from build123d import *

# Parameters (mm, degrees)
F0_W     = 127.9261372983
F0_H     = 87.7036768943
F1_DEPTH = 45.72
F2_R     = 17.7920916597
F3_DEPTH = 45.72
F4_W     = 127.9261372983
F4_H     = 45.72
F4_R     = 16.3569276355
F5_DEPTH = 130.048
F6_DEPTH = 25.4
F7_DEPTH = 104.394


with BuildPart() as f1:
    # F0 (on Top) → F1 (new body)
    with BuildSketch(Plane.XY):
        with Locations((-2.9164496809, -12.6540614292)):
            Rectangle(F0_W, F0_H)
    extrude(amount=F1_DEPTH)

    # F2 (on face) → F3 (cut)
    with BuildSketch(Plane.XY.offset(45.72)):
        with Locations((-40.4178053141, 0)):
            Circle(F2_R)
    extrude(amount=-F3_DEPTH, mode=Mode.SUBTRACT)

    # F4 (on face) → F5 (join)
    with BuildSketch(Plane(origin=(0, 31.197777018, 0), x_dir=(-1, 0, 0), z_dir=(0, 1, 0))):
        with Locations((2.9164496809, 22.86)):
            Rectangle(F4_W, F4_H)
        with Locations((14.2273971344, 27.2544236794)):
            Circle(F4_R, mode=Mode.SUBTRACT)
    extrude(amount=F5_DEPTH)

    # F6 (cut): a face of the model
    f6_faces = [f1.faces().sort_by_distance(p)[0] for p in [
        (-1.528037409, 54.3088302233, 0),
    ]]
    extrude(f6_faces, amount=-F6_DEPTH, mode=Mode.SUBTRACT)

    # F7 (add): a face of the model
    f7_faces = [f1.faces().sort_by_distance(p)[0] for p in [
        (58.5211311066, 52.3699385708, 25.4),
    ]]
    extrude(f7_faces, amount=F7_DEPTH)


solid = f1.part
Model file for the job. Use its own axes, mm. A direction names the side the tool comes from. Coordinates: 2 decimals unless noted, no trailing zeros. Order: outer loops, then holes, each group sorted by start corner. A loop starts at its lowest first (then second) coordinate and runs counter-clockwise, first axis right, second up. Notation, with made-up numbers: M 47,44.5 L 77,44.5 A24 cw 77,80.5 Z; hole C 68.25,75 d2. An arc over 180 degrees is marked long. Return JSON: item names as keys, results as strings.
1. Tool access for faces 1 (the face through (2.024, 97, -26)), 2 (the face through (12, 51, -78.994)), 3 (the face through (-14.613, 95.311, 43.607)): list every direction of +Z, -Z, +X, -X, +Y, -Y with a clear straight run to the whole face (end or side of a thin tool).
Ans:
{"face 1": "-Z, +Y", "face 2": "-Z, +X, -X, +Y, -Y", "face 3": "+Y"}
2. Drill centre lines: probe 1 along X at (y, z) = (50, -50.5); probe 2 along X at (y, z) = (5.5, -49); probe 3 along Y at (x, z) = (-30, -42.5). Where is each one in solid material? Low to high.
Ans:
{"probe 1": "-66.88 to -30.48, 2.02 to 61.05", "probe 2": "-66.88 to -57.34, -23.5 to 61.05", "probe 3": "-56.51 to -14.42, 14.42 to 31.2"}
3. Saw through at B-B (z = 14). Give the cut face in (x, y), and give its area (3 significant figures).
Ans:
{"outline": "M -66.88,-56.51 L 61.05,-56.51 L 61.05,161.25 L 2.02,161.25 L 2.02,31.2 L -30.48,31.2 L -30.48,161.25 L -66.88,161.25 Z; hole C -40.42,0 d35.58", "area": "22,600 mm^2"}
4. Saw through at D-D (x = -40). Give the cut face in (y, z).
Ans:
{"outline": "M -56.51,-78.99 L -17.79,-78.99 L -17.79,45.72 L -56.51,45.72 Z; M 17.79,-78.99 L 161.25,-78.99 L 161.25,45.72 L 17.79,45.72 Z"}
5. Pull direction Y, two halves, no side cores. Call faces 4 (the face through (-4, -56.506, -16)), 5 (the face through (-23.447, 5.344, -15.764)), 6 (the face through (-2, 51, 45.72)), 7 (the face through (-14, 31.198, -17)): +Y half, -Y half, draft (parallel to the pull), parting line (faces both ways), or undercut.
Ans:
{"face 4": "-Y half", "face 5": "undercut", "face 6": "draft", "face 7": "+Y half"}
6. Saw through at C-C (y = 92). Give the cut face in (x, z), and give its area (3 significant figures).
Ans:
{"outline": "M -66.88,-78.99 L -30.48,-78.99 L -30.48,25.4 A16.36 cw long 2.02,25.4 L 2.02,-78.99 L 61.05,-78.99 L 61.05,45.72 L -66.88,45.72 Z", "area": "12,100 mm^2"}
7. Flat gauge pins, fed straight in: pin 1 (4 mm diameter, centred on x = -22, y = 94, fed in from -Z); pin 2 (4 mm diameter, centred on x = -9, z = -37, fed in from +Y). Where does each tip first touch, or does it go through?
Ans:
{"pin 1": "z = 40.37", "pin 2": "y = 31.2"}
8. Saw through at A-A (y = 0). Give the cut face in (x, z).
Ans:
{"outline": "M -66.88,-78.99 L -58.21,-78.99 L -58.21,45.72 L -66.88,45.72 Z; M -22.63,-78.99 L 61.05,-78.99 L 61.05,45.72 L -22.63,45.72 Z"}
